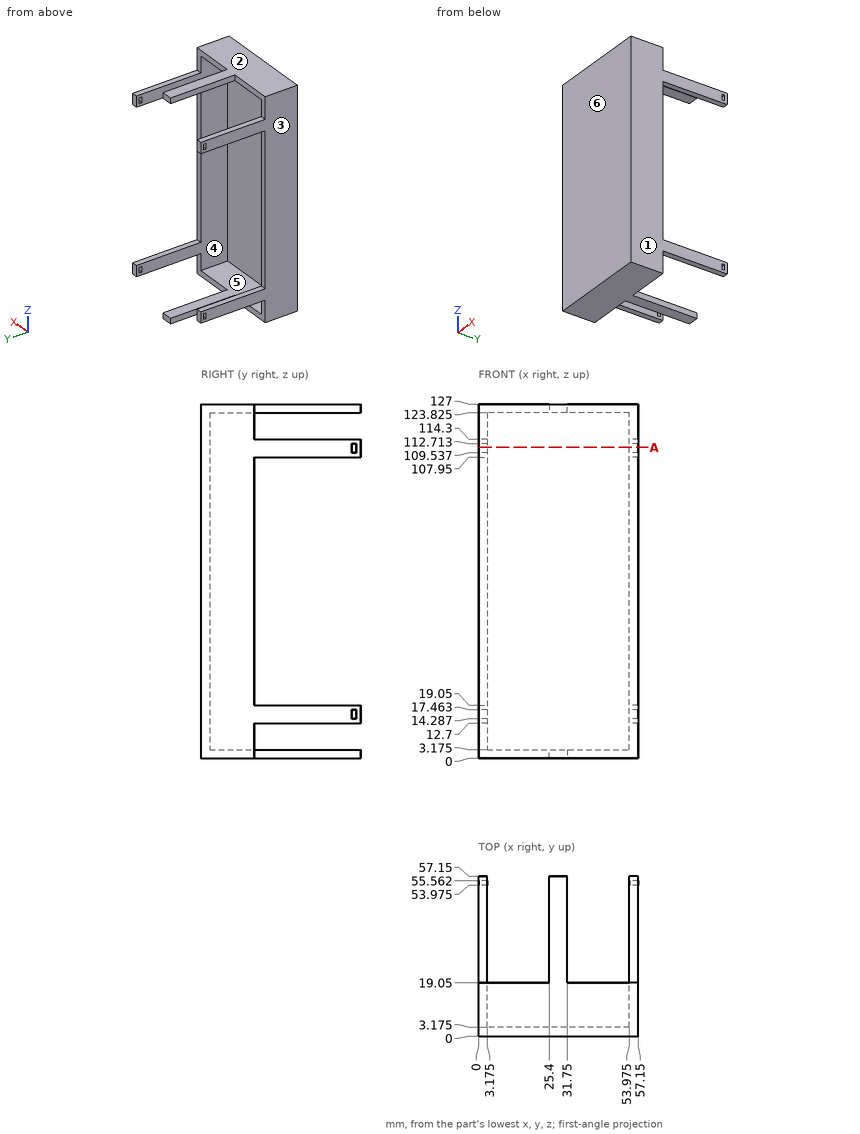
Input: dimensioned drawing with shaded views. Units: mm. Origin: part minimum x, y, z. A direction names the side the tool comes from. Round coordinates to 2 decimals unless told otherwise and drop trailing zeros.
Q1. Access query for the marked faces 5 and 6. Directions: +Z, -Z, +X, -X, +Y, -Y. A direction counts if a zero-diameter tool reaches every point of the face in a straight line with its end or side. Return the directions, or none.
Result sheet:
face 5: +Y
face 6: +Z, -Z, +X, -X, -Y
Q2. Mould query, pull axis X, two halves, no side actions, for the marked faces 1, 2, 3 and 4. Classes: released by +X, released by -X, zero draft, split by the parting line, or undercut.
Result sheet:
face 1: released by +X
face 2: zero draft
face 3: released by -X
face 4: undercut
Q3. Material intervals for probe 1 along Z at (x, y) = (25, 10) (1 decimal); probe 2 along Z at (x, y) = (3, 25); probe 3 along Y at (x, z) = (33.5, 43) (1 decimal), sorted ascending.
Result sheet:
probe 1: z = 0 to 3.2, 123.8 to 127
probe 2: z = 12.7 to 19.05, 107.95 to 114.3
probe 3: y = 0 to 3.2
Q4. Pin query (flat end, axial travel): pin 1 (1.3 mm diameter, centred on x = 1.5, y = 55, fed in from -Z); pin 2 (10 mm diameter, centred on x = 45.5, z = 4.5, fed in from +Y); pin 3 (1.7 mm diameter, centred on x = 1, y = 54.5, fed in from +Z). Return the tip coordinate at first contact, or that it passes through.
Result sheet:
pin 1: stops at z = 12.7
pin 2: stops at y = 19.05
pin 3: stops at z = 114.3
Q5. Section A-A, the plane z = 111.5. Give the number of separate pieces and of enclosed holes in the cut face, and give its area (3 significant figures).
Result sheet:
separate pieces: 3
enclosed holes: 0
area: 514 mm2
